from build123d import *

# Parameters (mm, degrees)
CIRPATTERN1_COUNT                = 12
CIRPATTERN2_COUNT                = 6
F_1_8_0_125_DIAMETER_HOLE1_D     = 3.175
F_1_8_0_125_DIAMETER_HOLE1_DEPTH = 3.175
F_1_8_0_125_DIAMETER_HOLE1_TIP   = 0.953866233


with BuildPart() as part:
    # Sketch1 → Revolve1 (revolve)
    with BuildSketch(Plane.XY):
        Polygon((-6.35, 0), (-88.9, 0), (-88.9, 12.7), (-50.8, 12.7), (-31.75, 31.75), (-6.35, 31.75), align=None)
    revolve(axis=Axis((0, 0, 0), (0, 1, 0)))

    # Sketch3 → 5/16 (0.3125) Diameter Hole1 (revolve, cut)
    with BuildSketch(Plane(origin=(76.2, 12.7, 0), x_dir=(0, 0, 1), z_dir=(1, 0, 0))):
        Polygon((0, 0), (0, 31.086665582), (3.96875, 28.702), (3.96875, 0), align=None)
    f_5_16_0_3125_diameter_hole1 = revolve(axis=Axis((76.2, 19.05, 0), (0, -1, 0)), mode=Mode.SUBTRACT)

    # CirPattern1: 5/16 (0.3125) Diameter Hole1 ×12 about axis
    cirpattern1_axis = Axis((0, 0, 0), (0, 1, 0))
    for i in range(1, CIRPATTERN1_COUNT):
        add(f_5_16_0_3125_diameter_hole1.rotate(cirpattern1_axis, i * 360 / CIRPATTERN1_COUNT), mode=Mode.SUBTRACT)

    # Sketch5 → 1/2 NPT Tapped Hole1 (revolve, cut)
    with BuildSketch(Plane(origin=(41.852788136, 21.647211864, 0), x_dir=(-0.707106781, 0.707106781, 0), z_dir=(0, 0, 1))):
        Polygon((0, 0), (0, 33.939543693), (8.9281, 28.575), (8.9281, 13.462), (9.479726792, 13.462), (9.8827971, 0), align=None)
    revolve(axis=Axis((46.342916197, 26.137339924, 0), (-0.707106781, -0.707106781, 0)), mode=Mode.SUBTRACT)

    # Sketch7 → 1/2 NPT Tapped Hole2 (revolve, cut)
    with BuildSketch(Plane(origin=(-41.852788136, 21.647211864, 0), x_dir=(-0.707106781, -0.707106781, 0), z_dir=(0, 0, 1))):
        Polygon((0, 0), (0, 34.066543693), (8.9281, 28.702), (8.9281, 13.462), (9.479726792, 13.462), (9.8827971, 0), align=None)
    revolve(axis=Axis((-46.342916197, 26.137339924, 0), (0.707106781, -0.707106781, 0)), mode=Mode.SUBTRACT)

    # Sketch9 → 1/4-20 Tapped Hole1 (revolve, cut)
    with BuildSketch(Plane(origin=(21.997045256, 31.75, -12.7), x_dir=(0, 0, 1), z_dir=(1, 0, 0))):
        Polygon((0, 0), (0, 18.043816902), (2.5527, 16.51), (2.5527, 0), align=None)
    f_1_4_20_tapped_hole1 = revolve(axis=Axis((21.997045256, 38.1, -12.7), (0, -1, 0)), mode=Mode.SUBTRACT)

    # CirPattern2: 1/4-20 Tapped Hole1 ×6 about axis
    cirpattern2_axis = Axis((0, 0, 0), (0, 1, 0))
    for i in range(1, CIRPATTERN2_COUNT):
        add(f_1_4_20_tapped_hole1.rotate(cirpattern2_axis, i * 360 / CIRPATTERN2_COUNT), mode=Mode.SUBTRACT)

    # 1/8 (0.125) Diameter Hole1
    with Locations(Plane(origin=(0, 0, 0), x_dir=(-1, 0, 0), z_dir=(0, -1, 0))):
        with Locations((35.745198541, -20.6375)):
            Hole(F_1_8_0_125_DIAMETER_HOLE1_D / 2, depth=F_1_8_0_125_DIAMETER_HOLE1_DEPTH)
            with Locations((0, 0, -(F_1_8_0_125_DIAMETER_HOLE1_DEPTH + F_1_8_0_125_DIAMETER_HOLE1_TIP / 2))):  # 118° drill point
                Cone(0, F_1_8_0_125_DIAMETER_HOLE1_D / 2, F_1_8_0_125_DIAMETER_HOLE1_TIP, mode=Mode.SUBTRACT)


solid = part.part
Can you work these out from the model? Positions are in its coordinate system, mm. A direction names the side the tool comes from. Give positions to 0.01 mm unless a question says otherwise; leave off trailing zeros. Order: outer loops, then holes, each group sorted by start corner. A loop starts at its lowest first (then second) coordinate and runs counter-clockwise, first axis right, second up. Notation, with made-up numbers: M 59,16 L 91,16 A30 cw 91,54 Z; hole C -8.75,-8.75 d2. An arc over 180 degrees is marked long. Use a Markdown table: item, result. Add a question column.
Item 1: Suppose I cut it at A-A (x = -76.2). List the corners of the cut face in (y, z) for me, then the cut area to 3 significant figures.
Item 2: For faces 4 (the cylindrical face through (19.845, 23.611, -11.328)), 5 (the cylindrical face through (-62.206, 6.439, 39.292)), which set-ups out of +Z, -Z, +X, -X, +Y, -Y let a thin tool reach every point of the face, with its end or its side?
Item 3: We'd pull the mould along X, two halves only. Please class faces 1 (the flat face through (-7, 31.75, 0)), 2 (the conical face through (-31.166, 30.825, 9.815)), 3 (the cylindrical face through (63.86, 6.44, -41.45)): +X half, -X half, draft (parallel to the pull), parting line (faces both ways), or undercut.
Item 4: Will these pins go through, and if not, where does the flat tip stop? pin 1 (1 mm diameter, centred on x = -31, y = 22, fed in from +Z); pin 2 (3.5 mm diameter, centred on x = -35.75, z = 20.64, fed in from +Y); pin 3 (6 mm diameter, centred on x = -61, y = 13.5, fed in from -Z); pin 4 (10 mm diameter, centred on x = 0, z = 0, fed in from -Y).
Item 5: Suppose I cut it at C-C (y = 26.5). Count the separate pieces of the cut face and the enclosed holes in it, then the cut area to 3 significant figures.
Item 6: If I drill on L1, parallel to Z at x = 0, y = 7; L2, parallel to X at y = 12.5, z = 5.5; L3, parallel to X at y = 22.5, z = -14, over which ranges is the centre line in solid material (lowest first)? Write a range as [from, to].
Item 7: Suppose I cut it at B-B (z = 76.2). List the corners of the cut face in (x, y) for me, then the cut area to 3 significant figures.
Answer sheet:
| question | item | result |
|---|---|---|
| 1 | outline | M 0,-45.79 L 12.7,-45.79 L 12.7,-3.97 L 0,-3.97 Z; M 0,3.97 L 12.7,3.97 L 12.7,45.79 L 0,45.79 Z |
| 1 | area | 1,060 mm² |
| 2 | face 4 | +Y |
| 2 | face 5 | +Y, -Y |
| 3 | face 1 | draft |
| 3 | face 2 | parting line |
| 3 | face 3 | undercut |
| 4 | pin 1 | stops at z = 28.52 |
| 4 | pin 2 | stops at y = 23.97 |
| 4 | pin 3 | stops at z = -67.28 |
| 4 | pin 4 | passes through |
| 5 | separate pieces | 1 |
| 5 | enclosed holes | 7 |
| 5 | area | 3,980 mm² |
| 6 | L1 | z = [-88.9, -80.17], [-72.23, -6.35], [6.35, 72.23], [80.17, 88.9] |
| 6 | L2 | x = [-88.73, -44.07], [-22.76, -3.17], [3.17, 22.76], [44.07, 88.73] |
| 6 | L3 | x = [-38.54, -24.19], [-19.8, 19.8], [24.19, 38.54] |
| 7 | outline | M -45.79,0 L -3.97,0 L -3.97,12.7 L -45.79,12.7 Z; M 3.97,0 L 45.79,0 L 45.79,12.7 L 3.97,12.7 Z |
| 7 | area | 1,060 mm² |
